Part model, mm, in its own coordinate system. Face numbers are marked on the shaded views. A direction names the side the tool comes from. Coordinates: 2 decimals unless noted, no trailing zeros. Loops run counter-clockwise (first coordinate to the right, second up) from the corner with the lowest first, then second, coordinate; pieces in that order, holes last.
Autodesk Inventor part; units mm, degrees
ref_plane "YZ Plane" through (0, 0, 0) normal (1, 0, 0) x (0, 1, 0)
ref_plane "XZ Plane" through (0, 0, 0) normal (0, 1, 0) x (-1, 0, 0)
ref_plane "XY Plane" through (0, 0, 0) normal (0, 0, 1) x (1, 0, 0)
sketch "Sketch1" plane through (0, 0, 0) normal (0, 0, 1) x (1, 0, 0)
  line L0 (12.7, 0) -> (12.7, 5.5)
  line L1 (0, 0) -> (12.7, 0)
  line L2 (12.7, 0) -> (12.7, 37.3027)
  line L3 (12.7, 37.3027) -> (0, 37.3027)
  line L4 (0, 37.3027) -> (0, 0)
  line L5 (6, 37.3027) -> (12.7, 33.4345)
  line L6 (6, 0) -> (12.7, 3.8682)
  circle A0 centre (6, 13.9014) radius 1.35
  circle A1 centre (6, 23.4014) radius 1.35
  line L7 (6, 23.4014) -> (6, 13.9014) construction
  line L8 (0, 0) -> (12.7, 7.3323)
  line L9 (12.7, 29.9704) -> (0, 37.3027)
  point P0 (6, 18.6514)
  point P1 (12.7, 18.6514)
  point P2 (12.7, 0)
  dimension "d2" = 9.5
  dimension "d3" = 2.7
  dimension "d4" = 2.7
  dimension "d15" = 37.3027
  dimension "d17" = 60
  dimension "d18" = 60
  dimension "d19" = 3
  dimension "d20" = 3
  dimension "d21" = 12.7
extrude "Extrusion1" add sketch "Sketch1" along normal blind 8 contours L6 L1 L8 L2 L0 | L4 L9 L2 L8 | L3 L5 L2 L9
extrude "Extrusion2" add sketch "Sketch1" against normal blind 6.35 and the other way blind 6 contours L6 L1 L8 L2 L0 | L3 L5 L2 L9
equation "\"d4\" = d3"
properties part number "Home Switch Mount X"
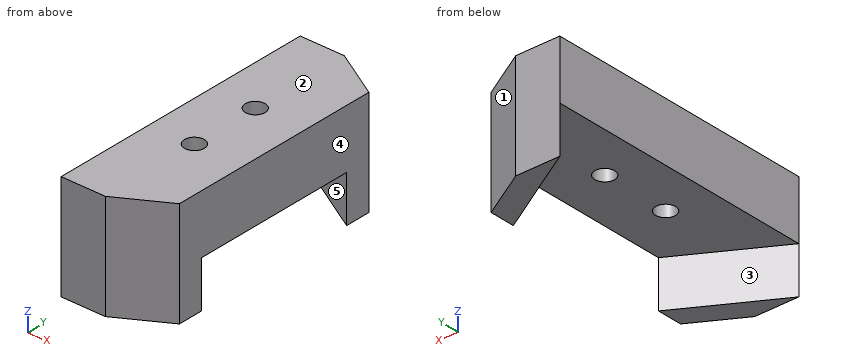
Q1. Saw through at C-C (x = 10). List the corners of the cut face in (y, z).
Q2. Mould opens along Y. For the marked faces 1, 2 and 3 say: released by +Y, released by -Y, zero draft, split by the parting line, or undercut.
Q3. Drop flat-ended pins along their axis: P1, Ø5, axis at x = 11, z = -1.5, coming from the -Y side; P2, Ø1, axis at x = 11, y = 27, coming from the -Z side. Give the stop position or say it passes through.
Q4. Saw through at B-B (y = 13). List the corners of the cut face in (x, z).
Q5. Probe line 1 (Y direction, x = 6, z = 5.5); line 2 (Y direction, x = 6.25, z = 3.75); line 3 (Z direction, x = 2, y = 25). List the from-to ranges inside material, lowest first.
Q6. Saw through at D-D (y = 29). List the corners of the cut face in (x, z), plus the area to 3 significant figures.
Q7. Saw through at A-A (z = -1). List the corners of the cut face in (x, y), plus the area to 3 significant figures.
Q8. Tool access for the marked faces 4 and 5: list every direction of +Z, -Z, +X, -X, +Y, -Y with a clear straight run to the whole face (end or side of a thin tool).
Checked values:
1. outline: (2.31, -6.35) - (5.77, -6.35) - (5.77, 0) - (31.53, 0) - (31.53, -6.35) - (34.99, -6.35) - (34.99, 8) - (2.31, 8) - close
2. face 1: released by +Y
2. face 2: zero draft
2. face 3: undercut
3. P1: stops at y = 1.44
3. P2: stops at z = 0
4. outline: (0, 0) - (5, 0) - (5, 8) - (0, 8) - close; (7, 0) - (12.7, 0) - (12.7, 8) - (7, 8) - close
5. line 1: y = 0 to 12.55, 15.25 to 22.05, 24.75 to 37.3
5. line 2: y = 0.14 to 12.57, 15.23 to 22.07, 24.73 to 37.16
5. line 3: z = 0 to 8
6. outline: (0, 0) - (12.7, 0) - (12.7, 8) - (0, 8) - close
6. area: 102 mm2
7. outline: (0, 0) - (6, 0) - (12.7, 3.87) - (12.7, 7.33) - close; (0, 37.3) - (12.7, 29.97) - (12.7, 33.43) - (6, 37.3) - close
7. area: 67.2 mm2
8. face 4: +Z, -Z, +X, +Y, -Y
8. face 5: -Z, -X
